Here's how the part is built. I have some questions about the finished solid (model axes, mm). A direction names the side the tool comes from. Round coordinates to 2 decimals unless told otherwise and drop trailing zeros. Loops run counter-clockwise (first coordinate to the right, second up) from the corner with the lowest first, then second, coordinate; pieces in that order, holes last. Notation, with made-up numbers: (-23, -16) - (-3, -16) arc R5 ccw to (-3, -8) - close; hole circle Ø8 at (50, -4.75). An arc over 180 degrees is marked (long way). Return JSON: item names as keys, results as strings. Group by question number.
```python
from build123d import *

# Parameters (mm, degrees)
SKETCH1_W           = 169.3418
SKETCH1_H           = 254
BOSS_EXTRUDE1_DEPTH = 45.72
SKETCH2_W           = 149.0218
SKETCH2_H           = 233.68
CUT_EXTRUDE1_DEPTH  = 40.64
CUT_EXTRUDE10_REACH = 310.679
F_12_PIN_MOUNT_R    = 2.7999944
CUT_EXTRUDE3_DEPTH  = 5.499989
CUT_EXTRUDE5_REACH  = 310.679
CUT_EXTRUDE6_START  = -254
CUT_EXTRUDE6_DEPTH  = 10.16
SKETCH6_R           = 2.7999944
CUT_EXTRUDE7_DEPTH  = 5.499989
CUT_EXTRUDE8_START  = -248.500011
SKETCH6_2_R         = 2.7999944
CUT_EXTRUDE8_DEPTH  = 5.499989
SKETCH7_R           = 5
BOSS_EXTRUDE2_DEPTH = 6.35
CUT_EXTRUDE9_START  = 6.35
SKETCH8_R           = 2.7999944
CUT_EXTRUDE9_DEPTH  = 5.499989


with BuildPart() as part:
    # Sketch1 → Boss-Extrude1 (new body)
    with BuildSketch(Plane(origin=(0, 0, 0), x_dir=(1, 0, 0), z_dir=(0, 1, 0))):
        with Locations((84.6709, 127)):
            Rectangle(SKETCH1_W, SKETCH1_H)
    extrude(amount=BOSS_EXTRUDE1_DEPTH)

    # Sketch2 → Cut-Extrude1 (cut)
    with BuildSketch(Plane(origin=(0, 45.72, 0), x_dir=(1, 0, 0), z_dir=(0, 1, 0))):
        with Locations((84.6709, 127)):
            Rectangle(SKETCH2_W, SKETCH2_H)
    extrude(amount=-CUT_EXTRUDE1_DEPTH, mode=Mode.SUBTRACT)

    # Cut-Sweep2: sweep along a path in Sketch3
    with BuildLine(Plane(origin=(0, 45.72, 0), x_dir=(1, 0, 0), z_dir=(0, 1, 0))) as cut_sweep2_path:
        Line((6.35, 11.43), (6.35, 242.57))
        ThreePointArc((6.35, 242.57), (7.837897552, 246.162102448), (11.43, 247.65))
        Line((11.43, 247.65), (157.9118, 247.65))
        ThreePointArc((157.9118, 247.65), (161.503902448, 246.162102448), (162.9918, 242.57))
        Line((162.9918, 242.57), (162.9918, 11.43))
        ThreePointArc((162.9918, 11.43), (161.503902448, 7.837897552), (157.9118, 6.35))
        Line((157.9118, 6.35), (11.43, 6.35))
        ThreePointArc((11.43, 6.35), (7.837897552, 7.837897552), (6.35, 11.43))
    # Sketch4 → Cut-Sweep2 (sweep, cut)
    with BuildSketch(Plane.XY.offset(-15.24)):
        Polygon((4.064, 45.72), (3.272383398, 43.942), (7.141616602, 43.942), (6.35, 45.72), align=None)
    sweep(path=cut_sweep2_path.line, mode=Mode.SUBTRACT)

    # Sketch13 → Cut-Extrude10 (cut, up to next)
    with BuildSketch(Plane(origin=(169.3418, 0, 0), x_dir=(0, 0, -1), z_dir=(1, 0, 0)), mode=Mode.PRIVATE) as cut_extrude10_sk1:
        with BuildLine():
            Line((48.5902, -10.7823), (48.5902, -12.4587))
            ThreePointArc((48.5902, -12.4587), (48.813384633, -12.997515367), (49.3522, -13.2207))
            Line((49.3522, -13.2207), (61.6458, -13.2207))
            ThreePointArc((61.6458, -13.2207), (62.184615367, -12.997515367), (62.4078, -12.4587))
            Line((62.4078, -12.4587), (62.4078, -10.7823))
            ThreePointArc((62.4078, -10.7823), (62.630984633, -10.243484633), (63.1698, -10.0203))
            Line((63.1698, -10.0203), (66.7004, -10.0203))
            ThreePointArc((66.7004, -10.0203), (69.771647593, -8.748147593), (71.0438, -5.6769))
            Line((71.0438, -5.6769), (71.0438, 2.1209))
            ThreePointArc((71.0438, 2.1209), (69.771647593, 5.192147593), (66.7004, 6.4643))
            Line((66.7004, 6.4643), (44.2976, 6.4643))
            ThreePointArc((44.2976, 6.4643), (41.226352407, 5.192147593), (39.9542, 2.1209))
            Line((39.9542, 2.1209), (39.9542, -5.6769))
            ThreePointArc((39.9542, -5.6769), (41.226352407, -8.748147593), (44.2976, -10.0203))
            Line((44.2976, -10.0203), (47.8282, -10.0203))
            ThreePointArc((47.8282, -10.0203), (48.367015367, -10.243484633), (48.5902, -10.7823))
        make_face()
    cut_extrude10_tool1 = extrude(cut_extrude10_sk1.sketch, amount=-CUT_EXTRUDE10_REACH, mode=Mode.PRIVATE) & part.part
    # Sketch13 → Cut-Extrude10 (cut, up to next)
    with BuildSketch(Plane(origin=(169.3418, 0, 0), x_dir=(0, 0, -1), z_dir=(1, 0, 0)), mode=Mode.PRIVATE) as cut_extrude10_sk2:
        with BuildLine():
            Line((191.5922, -10.7823), (191.5922, -12.4587))
            ThreePointArc((191.5922, -12.4587), (191.815384633, -12.997515367), (192.3542, -13.2207))
            Line((192.3542, -13.2207), (204.6478, -13.2207))
            ThreePointArc((204.6478, -13.2207), (205.186615367, -12.997515367), (205.4098, -12.4587))
            Line((205.4098, -12.4587), (205.4098, -10.7823))
            ThreePointArc((205.4098, -10.7823), (205.632984633, -10.243484633), (206.1718, -10.0203))
            Line((206.1718, -10.0203), (209.7024, -10.0203))
            ThreePointArc((209.7024, -10.0203), (212.773647593, -8.748147593), (214.0458, -5.6769))
            Line((214.0458, -5.6769), (214.0458, 2.1209))
            ThreePointArc((214.0458, 2.1209), (212.773647593, 5.192147593), (209.7024, 6.4643))
            Line((209.7024, 6.4643), (187.2996, 6.4643))
            ThreePointArc((187.2996, 6.4643), (184.228352407, 5.192147593), (182.9562, 2.1209))
            Line((182.9562, 2.1209), (182.9562, -5.6769))
            ThreePointArc((182.9562, -5.6769), (184.228352407, -8.748147593), (187.2996, -10.0203))
            Line((187.2996, -10.0203), (190.8302, -10.0203))
            ThreePointArc((190.8302, -10.0203), (191.369015367, -10.243484633), (191.5922, -10.7823))
        make_face()
    cut_extrude10_tool2 = extrude(cut_extrude10_sk2.sketch, amount=-CUT_EXTRUDE10_REACH, mode=Mode.PRIVATE) & part.part
    add(cut_extrude10_tool1.solids().sort_by_distance((169.3418, -2.58192, -55.499))[0], mode=Mode.SUBTRACT)
    add(cut_extrude10_tool2.solids().sort_by_distance((169.3418, -2.58192, -198.501))[0], mode=Mode.SUBTRACT)

    # 12 pin mount → Cut-Extrude3 (cut)
    with BuildSketch(Plane(origin=(169.3418, 0, 0), x_dir=(0, 0, -1), z_dir=(1, 0, 0))):
        with Locations((77.978, -13.716)):
            Circle(F_12_PIN_MOUNT_R)
        with Locations((77.978, 10.16)):
            Circle(F_12_PIN_MOUNT_R)
        with Locations((33.02, 10.16)):
            Circle(F_12_PIN_MOUNT_R)
        with Locations((33.02, -13.716)):
            Circle(F_12_PIN_MOUNT_R)
        with Locations((176.022, -13.716)):
            Circle(F_12_PIN_MOUNT_R)
        with Locations((220.98, -13.716)):
            Circle(F_12_PIN_MOUNT_R)
        with Locations((220.98, 10.16)):
            Circle(F_12_PIN_MOUNT_R)
        with Locations((176.022, 10.16)):
            Circle(F_12_PIN_MOUNT_R)
    extrude(amount=-CUT_EXTRUDE3_DEPTH, mode=Mode.SUBTRACT)

    # 4 pin connector → Cut-Extrude5 (cut, up to next)
    with BuildSketch(Plane.XY, mode=Mode.PRIVATE) as cut_extrude5_sk1:
        with BuildLine():
            Line((32.6263, 31.877), (47.1043, 31.877))
            ThreePointArc((47.1043, 31.877), (49.798376836, 30.761076836), (50.9143, 28.067))
            Line((50.9143, 28.067), (50.9143, 14.7066))
            ThreePointArc((50.9143, 14.7066), (49.798376836, 12.012523164), (47.1043, 10.8966))
            Line((47.1043, 10.8966), (32.6263, 10.8966))
            ThreePointArc((32.6263, 10.8966), (29.932223164, 12.012523164), (28.8163, 14.7066))
            Line((28.8163, 14.7066), (28.8163, 28.067))
            ThreePointArc((28.8163, 28.067), (29.932223164, 30.761076836), (32.6263, 31.877))
        make_face()
    cut_extrude5_tool1 = extrude(cut_extrude5_sk1.sketch, amount=-CUT_EXTRUDE5_REACH, mode=Mode.PRIVATE) & part.part
    add(cut_extrude5_tool1.solids().sort_by_distance((39.8653, 21.3868, 0))[0], mode=Mode.SUBTRACT)

    # Sketch5<2> → Cut-Extrude6 (cut)
    with BuildSketch(Plane.XY.offset(CUT_EXTRUDE6_START)):
        with BuildLine():
            Line((32.6263, 31.877), (47.1043, 31.877))
            ThreePointArc((47.1043, 31.877), (49.798376836, 30.761076836), (50.9143, 28.067))
            Line((50.9143, 28.067), (50.9143, 14.7066))
            ThreePointArc((50.9143, 14.7066), (49.798376836, 12.012523164), (47.1043, 10.8966))
            Line((47.1043, 10.8966), (32.6263, 10.8966))
            ThreePointArc((32.6263, 10.8966), (29.932223164, 12.012523164), (28.8163, 14.7066))
            Line((28.8163, 14.7066), (28.8163, 28.067))
            ThreePointArc((28.8163, 28.067), (29.932223164, 30.761076836), (32.6263, 31.877))
        make_face()
    extrude(amount=CUT_EXTRUDE6_DEPTH, mode=Mode.SUBTRACT)

    # Sketch6 → Cut-Extrude7 (cut)
    with BuildSketch(Plane.XY):
        with Locations((55.0418, 32.6136)):
            Circle(SKETCH6_R)
        with Locations((55.0418, 10.16)):
            Circle(SKETCH6_R)
        with Locations((24.6888, 10.16)):
            Circle(SKETCH6_R)
        with Locations((24.6888, 32.6136)):
            Circle(SKETCH6_R)
    extrude(amount=-CUT_EXTRUDE7_DEPTH, mode=Mode.SUBTRACT)

    # Sketch6<2> → Cut-Extrude8 (cut)
    with BuildSketch(Plane.XY.offset(CUT_EXTRUDE8_START)):
        with Locations((55.0418, 32.6136)):
            Circle(SKETCH6_2_R)
        with Locations((55.0418, 10.16)):
            Circle(SKETCH6_2_R)
        with Locations((24.6888, 10.16)):
            Circle(SKETCH6_2_R)
        with Locations((24.6888, 32.6136)):
            Circle(SKETCH6_2_R)
    extrude(amount=-CUT_EXTRUDE8_DEPTH, mode=Mode.SUBTRACT)

    # Sketch7 → Boss-Extrude2 (add)
    with BuildSketch(Plane(origin=(0, 5.08, 0), x_dir=(1, 0, 0), z_dir=(0, 1, 0))):
        with Locations(Location((55.4218, 82.485, 0), (0, 0, 90))):
            Circle(SKETCH7_R)
        with Locations(Location((121.0818, 82.485, 0), (0, 0, 90))):
            Circle(SKETCH7_R)
        with Locations(Location((121.0818, 171.515, 0), (0, 0, 90))):
            Circle(SKETCH7_R)
        with Locations(Location((55.4218, 171.515, 0), (0, 0, 90))):
            Circle(SKETCH7_R)
    extrude(amount=BOSS_EXTRUDE2_DEPTH)

    # Sketch8 → Cut-Extrude9 (cut)
    with BuildSketch(Plane(origin=(0, 5.08, 0), x_dir=(1, 0, 0), z_dir=(0, 1, 0)).offset(CUT_EXTRUDE9_START)):
        with Locations(Location((55.4218, 171.515, 0), (0, 0, 270))):
            Circle(SKETCH8_R)
        with Locations(Location((121.0818, 171.515, 0), (0, 0, 270))):
            Circle(SKETCH8_R)
        with Locations(Location((121.0818, 82.485, 0), (0, 0, 270))):
            Circle(SKETCH8_R)
        with Locations(Location((55.4218, 82.485, 0), (0, 0, 270))):
            Circle(SKETCH8_R)
    extrude(amount=-CUT_EXTRUDE9_DEPTH, mode=Mode.SUBTRACT)


solid = part.part
```
Q1. Imagine slicing it at B-B, the plane x = 99.5. List the corners of the cut face in (y, z) for me, and give its area (3 significant figures).
Q2. Please list where these lines run through material, in increasing order: line 1 (Z direction, x = 18.5, y = 28.5); line 2 (X direction, y = 29.5, z = -36); line 3 (Z direction, x = 27, y = 9.5).
Q3. For faces 1 (the conical face through (163.4, 45.02, -6.06)), 2 (the cylindrical face through (56.547, 34.975, -251.212)), 3 (the flat face through (40, 31.877, -5)), 4 (the flat face through (123, 11.43, -174)), which set-ups out of +Z, -Z, +X, -X, +Y, -Y let a thin tool reach every point of the face, with its end or its side?
Q4. Imagine slicing it at D-D, the plane y = 40. List the corners of the cut face in (x, z) for me, and give its area (3 significant figures).
Q5. Imagine slicing it at A-A, the plane y = 21. List the corners of the cut face in (x, z) for me.
Q6. If we mould it in two halves opening along Z, with no side actions, what happens to faces 5 (the flat face through (55, 10, -248.5)), 6 (the flat face through (83, 23, 0)), 7 (the flat face through (84, 26, -243.84)), 8 (the flat face through (28.816, 21, -249))? For each: +Z half, -Z half, draft (parallel to the pull), parting line (faces both ways), or undercut.
Q7. Imagine slicing it at C-C, the plane z = -63.5. List the corners of the cut face in (x, y) for me.
Q8. Will these pins go through, and if not, where does the flat tip stop? pin 1 Ø15.5 at (x, z) = (85, -230) entering from +Y; pin 2 Ø3 at (x, y) = (55, 11) entering from +Z; pin 3 Ø3 at (x, z) = (6.5, -61) entering from -Y.
Output values:
{
 "1": {"outline": "(0, -254) - (45.72, -254) - (45.72, -249.94) - (43.94, -250.73) - (43.94, -246.86) - (45.72, -247.65) - (45.72, -243.84) - (5.08, -243.84) - (5.08, -212.88) arc R4.34 cw to (2.12, -214.05) - (0, -214.05) - close; (0, -182.96) - (2.12, -182.96) arc R4.34 cw to (5.08, -184.12) - (5.08, -69.88) arc R4.34 cw to (2.12, -71.04) - (0, -71.04) - close; (0, -39.95) - (2.12, -39.95) arc R4.34 cw to (5.08, -41.12) - (5.08, -10.16) - (45.72, -10.16) - (45.72, -6.35) - (43.94, -7.14) - (43.94, -3.27) - (45.72, -4.06) - (45.72, 0) - (0, 0) - close", "area": "1,790 mm^2"},
 "2": {"line 1": "z = -254 to -243.84, -10.16 to 0", "line 2": "x = 0 to 10.16, 159.18 to 169.34", "line 3": "z = -248.5 to -243.84, -10.16 to -5.5"},
 "3": {"face 1": "none", "face 2": "-Z", "face 3": "+Z, -Z", "face 4": "+Y"},
 "4": {"outline": "(0, -254) - (169.34, -254) - (169.34, 0) - (0, 0) - close; hole (10.16, -243.84) - (159.18, -243.84) - (159.18, -10.16) - (10.16, -10.16) - close", "area": "8,190 mm^2"},
 "5": {"outline": "(0, -254) - (28.82, -254) - (28.82, -243.84) - (10.16, -243.84) - (10.16, -10.16) - (28.82, -10.16) - (28.82, 0) - (0, 0) - close; (50.91, -254) - (169.34, -254) - (169.34, 0) - (50.91, 0) - (50.91, -10.16) - (159.18, -10.16) - (159.18, -243.84) - (50.91, -243.84) - close"},
 "6": {"face 5": "-Z half", "face 6": "+Z half", "face 7": "undercut", "face 8": "draft"},
 "7": {"outline": "(0, 6.46) - (10.16, 6.46) - (10.16, 45.72) - (6.35, 45.72) - (7.14, 43.94) - (3.27, 43.94) - (4.06, 45.72) - (0, 45.72) - close; (159.18, 6.46) - (169.34, 6.46) - (169.34, 45.72) - (165.28, 45.72) - (166.07, 43.94) - (162.2, 43.94) - (162.99, 45.72) - (159.18, 45.72) - close"},
 "8": {"pin 1": "stops at y = 5.08", "pin 2": "stops at z = -5.5", "pin 3": "stops at y = 6.46"}
}
